from build123d import *

# Parameters (mm, degrees)
BOSS_EXTRUDE1_DEPTH = 25.4
SKETCH2_W           = 11.199999952
SKETCH2_H           = 23.399999936
SKETCH2_H_2         = 5.599999976
CUT_EXTRUDE1_DEPTH  = 48.558347416
BOSS_EXTRUDE2_DEPTH = 3.302
SKETCH4_W           = 3.175
SKETCH4_H           = 2.199999918
CUT_EXTRUDE2_DEPTH  = 8.024999952


with BuildPart() as part:
    # Sketch1 → Boss-Extrude1 (new, symmetric)
    with BuildSketch(Plane.XY):
        Polygon((0, 0), (8.024999952, 0), (8.024999952, -2.199999918), (-39.600000048, -2.199999918), (-39.600000048, -4.581249918), (11.199999952, -4.581249918), (11.199999952, 2.38125), (0, 2.38125), align=None)
    extrude(amount=BOSS_EXTRUDE1_DEPTH, both=True)

    # Sketch2 → Cut-Extrude1 (cut, through all)
    with BuildSketch(Plane(origin=(0, 2.38125, 0), x_dir=(1, 0, 0), z_dir=(0, 1, 0))):
        with Locations((5.599999976, 0)):
            Rectangle(SKETCH2_W, SKETCH2_H)
        with Locations((5.599999976, 14.499999956)):
            Rectangle(SKETCH2_W, SKETCH2_H_2)
    extrude(amount=-CUT_EXTRUDE1_DEPTH, mode=Mode.SUBTRACT)

    # Sketch3 → Boss-Extrude2 (add)
    with BuildSketch(Plane.ZY.offset(-11.199999952)):
        Polygon((22.89999992, 0), (19.72499992, 0), (19.72499992, -2.199999918), (11.699999968, -2.199999918), (11.699999968, -4.581249918), (22.89999992, -4.581249918), align=None)
        Polygon((11.699999968, 2.38125), (11.699999968, 0), (19.72499992, 0), (22.89999992, 0), (22.89999992, 2.38125), align=None)
    extrude(amount=-BOSS_EXTRUDE2_DEPTH)

    # Sketch4 → Cut-Extrude2 (cut)
    with BuildSketch(Plane(origin=(0, 0, 11.699999968), x_dir=(-1, 0, 0), z_dir=(0, 0, -1))):
        with Locations((-9.612499952, -1.099999959)):
            Rectangle(SKETCH4_W, SKETCH4_H)
    extrude(amount=-CUT_EXTRUDE2_DEPTH, mode=Mode.SUBTRACT)


solid = part.part
Check sheet for the modelled part. Datum: model origin and axes. Units: mm. A direction names the side the tool comes from. Give positions to 0.01 mm unless a question says otherwise; leave off trailing zeros. Loops run counter-clockwise (first coordinate to the right, second up) from the corner with the lowest first, then second, coordinate; pieces in that order, holes last. Notation, with made-up numbers: M 60,84 L 79,84 A29 ccw 79,105 Z; hole C -13.75,75 d1. An arc over 180 degrees is marked long. Use a Markdown table: item, result. Add a question column.
Q1. Scan lines: line 1 along Z through (x, y) = (4.5, 1); line 2 along X through (y, z) = (-1, 23) (3 decimals); line 3 along X through (y, z) = (-2.25, -12). Record each from-to range of solid material in increasing order. Write a range as [from, to].
Q2. Tool access check on faces 1 (the flat face through (7, 1, 11.7)), 2 (the flat face through (0, -3, -3)), 3 (the flat face through (0, 1, 19)), 4 (the flat face through (11.2, -1, -21)). Record the directions out of +Z, -Z, +X, -X, +Y, -Y that give a thin tool (end or side, any length) a straight path to the whole face; none if there is none.
Q3. Sectioned sample at A-A, the plane z = 17. Record the cut outline in (x, y), then the cut area to 3 significant figures.
Q4. Sectioned sample at B-B, the plane y = 1.5. Record the cut outline in (x, z), then the cut area to 3 significant figures.
Q5. Sectioned sample at D-D, the plane z = -10. Record the cut outline in (x, y).
Q6. Mould release check, pull along Y, two halves, no side actions. Record for faces 5 (the flat face through (6, 0, 17)), 6 (the flat face through (6, 2.381, -21)), 7 (the flat face through (-39.6, -3, 0)), 8 (the flat face through (4, 0, -21)): pulls with the +Y half, pulls with the -Y half, needs draft (parallel to the pull), parting line crosses it, or undercut.
Q7. Sectioned sample at C-C, the plane y = -3. Record the cut outline in (x, z), then the cut area to 3 significant figures.
Q8. Go/stop test with flat-tipped pins: pin 1 (3.5 mm diameter, centred on y = -1.5, z = -22.5, fed in from +X); pin 2 (2.5 mm diameter, centred on y = 2, z = -21.5, fed in from -X); pin 3 (1 mm diameter, centred on x = 13.5, y = -1, fed in from +Z). Record where each tip stops, or that it passes through.
Verdict:
| question | item | result |
|---|---|---|
| 1 | line 1 | [-25.4, -17.3], [11.7, 25.4] |
| 1 | line 2 | [8.025, 11.2] |
| 1 | line 3 | [-39.6, 0] |
| 2 | face 1 | +X, -X, +Y, -Y |
| 2 | face 2 | +X, +Y, -Y |
| 2 | face 3 | +Z, -Z, -X, +Y |
| 2 | face 4 | -Z, +X, +Y, -Y |
| 3 | outline | M -39.6,-4.58 L 14.5,-4.58 L 14.5,-2.2 L -39.6,-2.2 Z; M 0,0 L 14.5,0 L 14.5,2.38 L 0,2.38 Z |
| 3 | area | 163 mm^2 |
| 4 | outline | M 0,-25.4 L 11.2,-25.4 L 11.2,-17.3 L 0,-17.3 Z; M 0,11.7 L 14.5,11.7 L 14.5,22.9 L 11.2,22.9 L 11.2,25.4 L 0,25.4 Z |
| 4 | area | 281 mm^2 |
| 5 | outline | M -39.6,-4.58 L 0,-4.58 L 0,-2.2 L -39.6,-2.2 Z |
| 6 | face 5 | undercut |
| 6 | face 6 | pulls with the +Y half |
| 6 | face 7 | needs draft |
| 6 | face 8 | undercut |
| 7 | outline | M -39.6,-25.4 L 11.2,-25.4 L 11.2,-17.3 L 0,-17.3 L 0,11.7 L 14.5,11.7 L 14.5,22.9 L 11.2,22.9 L 11.2,25.4 L -39.6,25.4 Z |
| 7 | area | 2,290 mm^2 |
| 8 | pin 1 | x = 11.2 |
| 8 | pin 2 | x = 0 |
| 8 | pin 3 | z = 22.9 |
